```python
from build123d import *

# Parameters (mm, degrees)
BOSS_EXTRUDE1_DEPTH      = 27
BOSS_EXTRUDE2_DEPTH      = 6
BOSS_EXTRUDE2_DEPTH_BACK = 14
SKETCH2_R                = 20
BOSS_EXTRUDE3_START      = -6
BOSS_EXTRUDE3_DEPTH      = 14
BOSS_EXTRUDE4_START      = -14
BOSS_EXTRUDE4_DEPTH      = 14
BOSS_EXTRUDE5_START      = -20
SKETCH5_R                = 20
BOSS_EXTRUDE5_DEPTH      = 20
HOLE1_D                  = 20
SKETCH8_W                = 52
SKETCH8_H                = 28
BOSS_EXTRUDE6_DEPTH      = 4
BOSS_EXTRUDE7_DEPTH      = 4
HOLE2_D                  = 12
LPATTERN1_COUNT          = 2
LPATTERN1_PITCH          = 59.3


with BuildPart() as part:
    # Sketch1 → Boss-Extrude1 (new, symmetric)
    with BuildSketch(Plane(origin=(0, 0, 0), x_dir=(0, 0, -1), z_dir=(1, 0, 0))):
        Polygon((0, 0), (0, 20), (128, 20), (128, 0), (83, 0), (83, 8), (28, 8), (28, 0), align=None)
    extrude(amount=BOSS_EXTRUDE1_DEPTH, both=True)



with BuildPart() as body_2:
    # Sketch2 → Boss-Extrude2 (new, two sides: drawn at the far end of the back side and taken through both)
    with BuildSketch(Plane.XY.offset(-BOSS_EXTRUDE2_DEPTH_BACK)):
        with Locations((0, 70)):
            Circle(SKETCH2_R)
    extrude(amount=BOSS_EXTRUDE2_DEPTH + BOSS_EXTRUDE2_DEPTH_BACK)


with BuildPart() as part_1:
    add(part.part)

    add(body_2.part)  # Boss-Extrude3 merges body 2
    # Sketch3 → Boss-Extrude3 (add)
    with BuildSketch(Plane.XY.offset(6).offset(BOSS_EXTRUDE3_START)):
        with BuildLine():
            Line((27, 20), (-27, 20))
            Line((-27, 20), (-19.816768222, 72.70105484))
            ThreePointArc((-19.816768222, 72.70105484), (0, 50), (19.816768222, 72.70105484))
            Line((19.816768222, 72.70105484), (27, 20))
        make_face()
    extrude(amount=-BOSS_EXTRUDE3_DEPTH)

    # Sketch4 → Boss-Extrude4 (add)
    with BuildSketch(Plane.XY.offset(-66).offset(BOSS_EXTRUDE4_START)):
        with BuildLine():
            Line((-27, 20), (27, 20))
            Line((27, 20), (19.816768222, 72.70105484))
            ThreePointArc((19.816768222, 72.70105484), (0, 90), (-19.816768222, 72.70105484))
            Line((-19.816768222, 72.70105484), (-27, 20))
        make_face()
    extrude(amount=BOSS_EXTRUDE4_DEPTH)

    # Sketch5 → Boss-Extrude5 (add)
    with BuildSketch(Plane.XY.offset(-66).offset(BOSS_EXTRUDE5_START)):
        with Locations((0, 70)):
            Circle(SKETCH5_R)
    extrude(amount=BOSS_EXTRUDE5_DEPTH)

    # Hole1 (through all)
    with Locations(Plane.XY.offset(6)):
        with Locations((0, 70)):
            Hole(HOLE1_D / 2)

    # Sketch8 → Boss-Extrude6 (add, symmetric)
    with BuildSketch(Plane(origin=(0, 0, 0), x_dir=(0, 0, -1), z_dir=(1, 0, 0))):
        with Locations((40, 34)):
            Rectangle(SKETCH8_W, SKETCH8_H)
    extrude(amount=BOSS_EXTRUDE6_DEPTH, both=True)

    # Sketch9 → Boss-Extrude7 (add, symmetric)
    with BuildSketch(Plane(origin=(0, 0, 0), x_dir=(0, 0, -1), z_dir=(1, 0, 0))):
        Polygon((80, 48), (128, 20), (80, 20), align=None)
    extrude(amount=BOSS_EXTRUDE7_DEPTH, both=True)

    # Hole2 (through all)
    with Locations(Plane(origin=(0, 20, 0), x_dir=(1, 0, 0), z_dir=(0, 1, 0))):
        with Locations((18, 108), (-18, 108)):
            hole2 = Hole(HOLE2_D / 2)

    # LPattern1: Hole2 ×2
    with Locations(*[(0, 0, i * LPATTERN1_PITCH) for i in range(1, LPATTERN1_COUNT)]):
        add(hole2, mode=Mode.SUBTRACT)


solid = part_1.part
```
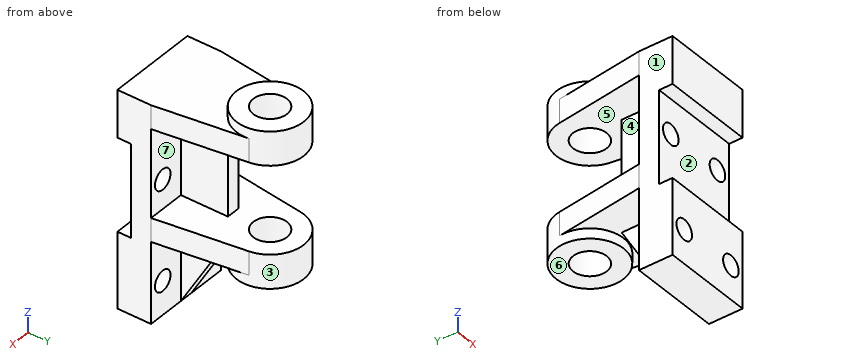
For this review, take the finished solid that the model builds, in its own axes (mm). Face numbers are marked on the shaded views. A direction names the side the tool comes from. Coordinates: 2 decimals unless noted, no trailing zeros. Loops run counter-clockwise (first coordinate to the right, second up) from the corner with the lowest first, then second, coordinate; pieces in that order, holes last. Notation, with made-up numbers: (-20.75, 51) -> (30.25, 51) arc R26 ccw to (30.25, 88) -> close; hole circle Ø3 at (-14.5, 4.5). An arc over 180 degrees is marked (long way). Return JSON: item names as keys, results as strings. Group by question number.
(1) Consider section D-D, the plane z = -20.5. Give the boundary of the cut face in (x, y), plus the area to 3 significant figures.
(2) Consider section C-C, the plane x = 0. Give the boundary of the cut face in (y, z).
(3) Tool access review of the marked faces 4, 5, 6 and 7: name each direction out of +Z, -Z, +X, -X, +Y, -Y from which nothing blocks a thin tool from reaching the whole face with its end or side.
(4) Mouldability with a two-part tool opening along Y and no side actions: class the marked faces 1, 2 and 3 as pulls with the +Y half, pulls with the -Y half, needs draft (parallel to the pull), parting line crosses it, or undercut.
(5) Consider section B-B, the plane z = -48.7. Give the boundary of the cut face in (x, y), plus the area to 3 significant figures.
(6) To check wall thickness, follow L1, parallel to Z at x = 18, y = 10.5; L2, parallel to X at y = 14, z = -108; L3, parallel to Z at x = 1.5, y = 58. State the ranges of each line that lie inside material, in increasing order.
(7) Consider section A-A, the plane y = 5. Give the boundary of the cut face in (x, z), plus the area to 3 significant figures.
(8) For pin 1 Ø11.5 at (x, z) = (12, -112.5) entering from +Y; pin 2 Ø14 at (y, z) = (34, -44.5) entering from +X; pin 3 Ø8 at (x, z) = (-10, -18) entering from -Y; pin 4 Ø1.5 at (x, z) = (-1, -73.5) entering from +Y, all flat-tipped, find the tip position at first contact; note any pin that passes through.
Results below:
{
 "1": {"outline": "(-27, 0) -> (27, 0) -> (27, 20) -> (4, 20) -> (4, 48) -> (-4, 48) -> (-4, 20) -> (-27, 20) -> close", "area": "1,300 mm2"},
 "2": {"outline": "(0, -128) -> (20, -128) -> (48, -80) -> (50, -80) -> (50, -86) -> (60, -86) -> (60, -66) -> (48, -66) -> (48, -14) -> (60, -14) -> (60, 6) -> (50, 6) -> (50, 0) -> (0, 0) -> (0, -28) -> (8, -28) -> (8, -83) -> (0, -83) -> close; (80, -86) -> (90, -86) -> (90, -66) -> (80, -66) -> close; (80, -14) -> (90, -14) -> (90, 6) -> (80, 6) -> close"},
 "3": {"face 4": "-X, +Y", "face 5": "+Y", "face 6": "-Z, +X, -X, +Y", "face 7": "+X, +Y"},
 "4": {"face 1": "needs draft", "face 2": "pulls with the -Y half", "face 3": "undercut"},
 "5": {"outline": "(-27, 8) -> (-24, 8) -> (-24, 20) -> (-27, 20) -> close; (-12, 8) -> (12, 8) -> (12, 20) -> (4, 20) -> (4, 48) -> (-4, 48) -> (-4, 20) -> (-12, 20) -> close; (24, 8) -> (27, 8) -> (27, 20) -> (24, 20) -> close", "area": "584 mm2"},
 "6": {"L1": "z = -128 to -114, -102 to -54.7, -42.7 to 0", "L2": "x = -27 to -24, -12 to 12, 24 to 27", "L3": "z = -86 to -66, -14 to 6"},
 "7": {"outline": "(-27, -128) -> (27, -128) -> (27, -83) -> (-27, -83) -> close; (-27, -28) -> (27, -28) -> (27, 0) -> (-27, 0) -> close; hole circle Ø12 at (-18, -108); hole circle Ø12 at (18, -108)", "area": "3,720 mm2"},
 "8": {"pin 1": "stops at y = 20", "pin 2": "stops at x = 4", "pin 3": "stops at y = 0", "pin 4": "stops at y = 90"}
}
